Verification items for the finished model (mm, model axes). Face numbers are marked on the shaded views. A direction names the side the tool comes from. Give positions to 0.01 mm unless a question says otherwise; leave off trailing zeros. Order: outer loops, then holes, each group sorted by start corner. A loop starts at its lowest first (then second) coordinate and runs counter-clockwise, first axis right, second up.
from build123d import *

# Parameters (mm, degrees)
F0_W     = 22
F0_H     = 35
F0_R     = 2.75
F1_DEPTH = 20
F2_R     = 5.5
F2_R_2   = 2.75
F3_DEPTH = 15
F5_DEPTH = 5
F7_DEPTH = 2.5


with BuildPart() as f1:
    # F0 (on Top) → F1 (new body)
    with BuildSketch(Plane.XY):
        with Locations((-11, -17.5)):
            Rectangle(F0_W, F0_H)
        with Locations((-11.25, -27.75)):
            Circle(F0_R, mode=Mode.SUBTRACT)
    extrude(amount=F1_DEPTH)

    # F2 (on face) → F3 (cut)
    with BuildSketch(Plane.XY.offset(20)):
        with Locations((-11.25, -27.75)):
            Circle(F2_R)
        with Locations((-11.25, -27.75)):
            Circle(F2_R_2, mode=Mode.SUBTRACT)
    extrude(amount=-F3_DEPTH, mode=Mode.SUBTRACT)

    # F4 (on face) → F5 (cut)
    with BuildSketch(Plane.XY.offset(20)):
        with BuildLine():
            Line((0, 0), (-22, 0))
            Line((-22, 0), (-22, -24.509916256))
            ThreePointArc((-22, -24.509916256), (-10.7524902947, -20.1460276214), (0, -14.6748347853))
            Line((0, -14.6748347853), (0, 0))
        make_face()
    extrude(amount=-F5_DEPTH, mode=Mode.SUBTRACT)

    # F6 (on face) → F7 (cut)
    with BuildSketch(Plane.XY.offset(15)):
        with BuildLine():
            Line((0, 0), (-22, 0))
            Line((-22, 0), (-22, -22.009916256))
            ThreePointArc((-22, -22.009916256), (-10.7298589355, -17.696651493), (0, -12.1748347853))
            Line((0, -12.1748347853), (0, 0))
        make_face()
    extrude(amount=-F7_DEPTH, mode=Mode.SUBTRACT)


solid = f1.part
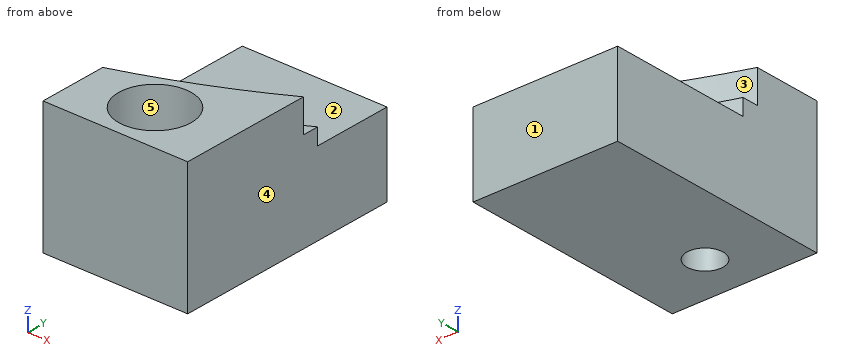
(1) Scan lines: line 1 (Y direction, x = -11.25, z = 3.1); line 2 (Y direction, x = -11.25, z = 11.25); line 3 (Z direction, x = -18.5, y = -16.5). Record each from-to range of solid material in increasing order.
Solved:
line 1: y = -35 to -30.5, -25 to 0
line 2: y = -35 to -33.25, -22.25 to 0
line 3: z = 0 to 12.5
(2) Section check A-A, the plane y = -27.75. Enter the section's corners in (x, z), then the cut area to 4 significant figures.
Solved:
outline: (-22, 0) - (-14, 0) - (-14, 5) - (-16.75, 5) - (-16.75, 20) - (-22, 20) - close; (-8.5, 0) - (0, 0) - (0, 20) - (-5.75, 20) - (-5.75, 5) - (-8.5, 5) - close
area: 247.5 mm2
(3) Release check for a two-part mould opening along Y. For the marked faces 3, 4 and 5 record: pulls with the +Y half, pulls with the -Y half, needs draft (parallel to the pull), parting line crosses it, or undercut.
Solved:
face 3: pulls with the +Y half
face 4: needs draft
face 5: undercut
(4) Section check B-B, the plane z = 2. Enter the section's corners in (x, y).
Solved:
outline: (-22, -35) - (0, -35) - (0, 0) - (-22, 0) - close; hole circle Ø5.5 at (-11.25, -27.75)
(5) Set-up check for the marked faces 1 and 2: record each of +Z, -Z, +X, -X, +Y, -Y from which the full face is reachable in a straight line by a thin tool's end or side.
Solved:
face 1: +Z, -Z, +X, -X, +Y
face 2: +Z, -X, +Y
(6) Go/stop test with flat-tipped pins: pin 1 (1 mm diameter, centred on x = -10.5, y = -27.5, fed in from +Z); pin 2 (9 mm diameter, centred on x = -11.25, y = -27.75, fed in from +Z); pin 3 (6.5 mm diameter, centred on x = -11.25, y = -27.75, fed in from -Z); pin 4 (3 mm diameter, centred on x = -9.5, z = 17.5, fed in from +Y). Record where each tip stops, or that it passes through.
Solved:
pin 1: passes through
pin 2: stops at z = 5
pin 3: stops at z = 0
pin 4: stops at y = -18.87
(7) Section check C-C, the plane x = -13.5. Enter the section's corners in (y, z), then the cut area to 3 significant figures.
Solved:
outline: (-35, 0) - (-29.33, 0) - (-29.33, 5) - (-32.77, 5) - (-32.77, 20) - (-35, 20) - close; (-26.17, 0) - (0, 0) - (0, 12.5) - (-18.89, 12.5) - (-18.89, 15) - (-21.33, 15) - (-21.33, 20) - (-22.73, 20) - (-22.73, 5) - (-26.17, 5) - close
area: 380 mm2
(8) Section check D-D, the plane y = -9. Enter the section's corners in (x, z).
Solved:
outline: (-22, 0) - (0, 0) - (0, 12.5) - (-22, 12.5) - close
